from build123d import *

# Parameters (mm, degrees)
F1_DEPTH = 25.4
F2_W     = 20.863877578
F2_H     = 13.4999741197
F3_DEPTH = 25.401
F4_W     = 7.9661535591
F4_H     = 12.7
F5_DEPTH = 25.4


with BuildPart() as f1:
    # F0 (on Front) → F1 (new body)
    with BuildSketch(Plane.XZ):
        Polygon((6.35, 0), (0, 0), (0, -25.4), (38.1, -25.4), (38.1, -12.7), (6.35, -12.7), align=None)
    extrude(amount=F1_DEPTH)

    # F2 (on Top) → F3 (cut, through all)
    with BuildSketch(Plane.XY):
        with Locations((28.710431435, -19.4499870598)):
            Rectangle(F2_W, F2_H)
    extrude(amount=-F3_DEPTH, mode=Mode.SUBTRACT)

    # F4 (on Right) → F5 (cut)
    with BuildSketch(Plane.YZ):
        with Locations((-23.0330767795, -6.35)):
            Rectangle(F4_W, F4_H)
    extrude(amount=F5_DEPTH, mode=Mode.SUBTRACT)


solid = f1.part
For this review, take the finished solid that the model builds, in its own axes (mm). A direction names the side the tool comes from. Round coordinates to 2 decimals unless told otherwise and drop trailing zeros. Write each loop counter-clockwise with the first axis right and the second up, starting at its lowest first coordinate (ties: lowest second). Pieces come first, ordered by that corner, then holes. Notation, with made-up numbers: (51.5, 70.25) - (68.5, 70.25) arc R17 ccw to (68.5, 96.25) - close; hole circle Ø5 at (86, 11.25). An arc over 180 degrees is marked (long way). Use a Markdown table: item, result.
Q1. We need section B-B (y = -8). Give the boundary of the cut face in (x, z), plus the area to 3 significant figures.
Derived:
| item | result |
|---|---|
| outline | (0, -25.4) - (38.1, -25.4) - (38.1, -12.7) - (6.35, -12.7) - (6.35, 0) - (0, 0) - close |
| area | 565 mm2 |
Q2. Machinability: for faces 1 (the flat face through (6.35, -9, -6)), 2 (the flat face through (3, -19.05, -6)), 3 (the flat face through (28, -12.7, -19)), 4 (the flat face through (15, 0, -18)), which of the approach directions +Z, -Z, +X, -X, +Y, -Y give a long, thin tool a straight path to every point of the face, cutting with its end or side? Answer none if there is none.
Derived:
| item | result |
|---|---|
| face 1 | +Z, +X, +Y, -Y |
| face 2 | +Z, +X, -X, -Y |
| face 3 | +Z, -Z, +X, -Y |
| face 4 | +Z, -Z, +X, -X, +Y |
Q3. We need section C-C (z = -9.75). Give the boundary of the cut face in (x, y).
Derived:
| item | result |
|---|---|
| outline | (0, -19.05) - (6.35, -19.05) - (6.35, 0) - (0, 0) - close |
Q4. We need section A-A (x = 4.5). Give the boundary of the cut face in (y, z), plus the area to 3 significant figures.
Derived:
| item | result |
|---|---|
| outline | (-25.4, -25.4) - (0, -25.4) - (0, 0) - (-19.05, 0) - (-19.05, -12.7) - (-25.4, -12.7) - close |
| area | 565 mm2 |
Q5. Clearance check with flat-ended pins moving along their axes: pin 1 (4 mm diameter, centred on y = -21, z = -20, fed in from +X); pin 2 (5 mm diameter, centred on x = 3.5, z = -7.5, fed in from -Y); pin 3 (14 mm diameter, centred on x = 25.5, z = -18, fed in from -Y). State where each tip first meets the part, or that it passes through.
Derived:
| item | result |
|---|---|
| pin 1 | stops at x = 18.28 |
| pin 2 | stops at y = -19.05 |
| pin 3 | stops at y = -12.7 |
Q6. We need section D-D (x = 23.5). Give the boundary of the cut face in (y, z), plus the area to 3 significant figures.
Derived:
| item | result |
|---|---|
| outline | (-12.7, -25.4) - (0, -25.4) - (0, -12.7) - (-12.7, -12.7) - close |
| area | 161 mm2 |
Q7. Wall thickness on line 1 along X through (y, z) = (-17.75, -16.75); line 2 along X through (y, z) = (-15.75, -10.25); line 3 along Y through (x, z) = (5, -11): over which ranges is each line inside the solid? List them lowest first.
Derived:
| item | result |
|---|---|
| line 1 | x = 0 to 18.28 |
| line 2 | x = 0 to 6.35 |
| line 3 | y = -19.05 to 0 |
